```python
from build123d import *

# Parameters (mm, degrees)
F0_R     = 63.5
F0_R_2   = 38.1
F1_DEPTH = 25.4
F2_R     = 12.69999
F3_R     = 12.69999


# Not quite as in the source:
# - a fillet or chamfer is up to 0.001 mm smaller than in the source, because OpenCascade refuses the exact size


with BuildPart() as f1:
    # F0 (on Front) → F1 (new body)
    with BuildSketch(Plane.XZ):
        Circle(F0_R)
        Circle(F0_R_2, mode=Mode.SUBTRACT)
    extrude(amount=F1_DEPTH)

    # F2 (radius 12.7 in the source; OpenCascade refuses exactly that, so slightly less here)
    f2_edges = [f1.edges().sort_by_distance(p)[0] for p in [
        (-38.1, -25.4, 0),
        (-38.1, 0, 0),
    ]]
    fillet(f2_edges, radius=F2_R)

    # F3 (radius 12.7 in the source; OpenCascade refuses exactly that, so slightly less here)
    f3_edges = [f1.edges().sort_by_distance(p)[0] for p in [
        (-63.5, -25.4, 0),
        (-63.5, 0, 0),
    ]]
    fillet(f3_edges, radius=F3_R)


solid = f1.part
```
Design review of the part built by this model. Coordinates are the model's own, in mm. Round coordinates to 2 decimals unless told otherwise and drop trailing zeros. Order: outer loops, then holes, each group sorted by start corner. A loop starts at its lowest first (then second) coordinate and runs counter-clockwise, first axis right, second up. Notation, with made-up numbers: (28.5, 26.5) - (48.5, 26.5) arc R23 cw to (48.5, 47.5) - close; hole circle Ø1 at (56.25, 5). An arc over 180 degrees is marked (long way). Return JSON: item names as keys, results as strings.
Q1. Wall thickness on L1, parallel to Z at x = 0, y = -12.7; L2, parallel to Z at x = 15, y = -23.25; L3, parallel to Y at x = 46, z = -19.5: over which ranges is each line inside the solid? List them lowest first. Write a range as [from, to].
Computed values:
{"L1": "z = [-63.5, -38.1], [38.1, 63.5]", "L2": "z = [-55.89, -41.08], [41.08, 55.89]", "L3": "y = [-25.37, -0.03]"}
Q2. Consider section C-C on y = -9.5. Write out the cut boundary in (x, z), plus the area to 3 significant figures.
Computed values:
{"outline": "circle Ø126.18 at (0, 0); hole circle Ø77.02 at (0, 0)", "area": "7,850 mm2"}
Q3. For pin 1 Ø3 at (x, y) = (-11.5, -15) entering from -Z; pin 2 Ø2 at (y, z) = (-21, 9) entering from +X; pin 3 Ø5 at (y, z) = (-16, -42) entering from -X, all flat-tipped, find the tip position at first contact; note any pin that passes through.
Computed values:
{"pin 1": "stops at z = -62.58", "pin 2": "stops at x = 60.54", "pin 3": "stops at x = -49.3"}
Q4. Consider section D-D on y = -18.75. Write out the cut boundary in (x, z).
Computed values:
{"outline": "circle Ø123.93 at (0, 0); hole circle Ø79.27 at (0, 0)"}
